Autodesk Inventor part; units mm, degrees
ref_plane "YZ Plane" through (0, 0, 0) normal (1, 0, 0) x (0, 1, 0)
ref_plane "XZ Plane" through (0, 0, 0) normal (0, 1, 0) x (-1, 0, 0)
ref_plane "XY Plane" through (0, 0, 0) normal (0, 0, 1) x (1, 0, 0)
sketch "Sketch1" plane through (0, 0, 0) normal (0, 0, 1) x (1, 0, 0)
  arc A0 (-97, -1740) -> (-70, 0) centre (-11100.8726, -699.0408) ccw
  line L0 (0, 0) -> (-70, 0)
  line L1 (0, -16.732) -> (-68.9524, -16.732) construction
  line L2 (0, -496.732) -> (-49.7243, -496.732) construction
  line L3 (0, -976.732) -> (-51.3615, -976.732) construction
  line L4 (0, -1456.732) -> (-73.8734, -1456.732) construction
  line L5 (-97, -1740) -> (0, -1740)
  line L6 (0, 0) -> (0, -1740)
  line L7 (0, -1730) -> (-10.3553, -1740)
  point P0 (-20, 0)
  dimension "d33" = 50
  dimension "d58" = 480
  dimension "d59" = 480
  dimension "d60" = 480
  dimension "d141" = 1740
  dimension "d148" = 70
  dimension "d149" = 11053
  dimension "d150" = 97
  dimension "d151" = 136
  dimension "d153" = 10
extrude "Plate3" add sketch "Sketch1" along normal blind 3 contours A0 L0 L6 L7 L5
sketch "Sketch3" plane through (-3, 0, 3) normal (1, 0, 0) x (0, 1, 0)
  line L0 (-1730, 0) -> (0, 0)
  line L1 (0, 0) -> (0, 20)
  line L2 (0, 20) -> (-1730, 20)
  line L3 (-1730, 20) -> (-1730, 0)
edge flange "Flange2" height 20 angle 90 thickness 3 bend radius 5 thickness toward (1, 0, 0) relief round relief width 3 relief depth 1.5 edges at (0, -865, 3) wall of the first edge with corners at (-3, -1730, 3) (-3, 0, 3) (-3, 0, -17) (-3, -1730, -17)
bend "Bend2"
corner "Corner2"
sketch "Sketch5" plane through (0, 0, 0) normal (0, 0, 1) x (1, 0, 0)
  line L0 (-8, -1737.7255) -> (-8, 0)
  line L1 (-70, 0) -> (-8, 0)
  arc A0 (-97, -1740) -> (-70, 0) centre (-11100.8726, -699.0408) ccw
  line L2 (0, 0) -> (0, -1730)
  line L3 (0, -198.9) -> (-28, -198.9)
  line L4 (0, -201.1) -> (-3, -201.1)
  line L5 (-3, -1730) -> (-3, 0)
  line L6 (-28, -198.9) -> (-28, -201.1)
  line L7 (0, -608.9) -> (-48.2402, -608.9) construction
  line L8 (0, -1018.9) -> (-52.5018, -1018.9) construction
  line L9 (0, -1428.9) -> (-71.9962, -1428.9) construction
  line L10 (-10.3553, -1740) -> (-97, -1740)
  line L11 (0, -198.9) -> (0, -218.9)
  line L12 (-3, -198.9) -> (-3, -201.1) construction
  line L13 (0, -218.9) -> (-3, -218.9)
  line L14 (-28, -198.9) -> (-59.1939, -198.9) construction
  line L15 (-28, -201.1) -> (-59.0945, -201.1) construction
  line L16 (-3, -201.1) -> (-3, -218.9)
  line L17 (-3, -201.1) -> (-28, -201.1)
  line L18 (-3, -218.9) -> (-8, -218.9)
  line L19 (-8, -1737.7255) -> (-10.3553, -1740)
  line L20 (-4.4351, -201.1) -> (0, -205.5351)
  line L21 (-4.4351, -201.1) -> (1.8371, -201.1) construction
  line L22 (-10.3553, -1740) -> (-10.3553, -1770)
  point P0 (0, 0)
  point P1 (845.25, -380.4205)
  point P2 (848, -380.4205)
  point P3 (-28, -200)
  point P4 (850, -410.4205)
  point P5 (-3, -198.9)
  point P6 (-3, -218.9)
  point P7 (-8, -201.1)
  point P8 (0, -205.5351)
  dimension "d69" = 1730
  dimension "d70" = 2.2
  dimension "d76" = 59.1939
  dimension "d80" = 48.2402
  dimension "d102" = 71.9962
  dimension "d104" = 52.5018
  dimension "d106" = 3
  dimension "d107" = 20
  dimension "d108" = 200
  dimension "d112" = 28
  dimension "d142" = 410
  dimension "d143" = 410
  dimension "d144" = 410
  dimension "d154" = 45
  dimension "d155" = 30
  dimension "d156" = 341.1
extrude "Extrusion2" cut sketch "Sketch5" along normal through all both and the other way through all contours L17 L6 L3 L0 | L0 L3 L5 L17 | L17 L5 L20 | L5 L4 L2 L20 | L3 L2 L4 L5
pattern_linear "Rectangular Pattern3" count 4 spacing 410 along (0, -1, 0) of "Extrusion2"
sketch "Sketch7" plane through (0, 0, 0) normal (0, 0, 1) x (1, 0, 0)
  line L0 (0, 0) -> (0, -198.9)
  line L1 (0, 0) -> (-100, 0)
  line L2 (-100, 0) -> (-100, -940)
  line L3 (-100, -940) -> (0, -940)
  line L4 (0, -940) -> (0, 0)
  line L5 (-100, -1740) -> (0, -1740)
  line L6 (0, -1740) -> (0, -940)
  line L7 (0, -940) -> (-100, -940)
  line L8 (-100, -940) -> (-100, -1740)
  line L9 (-97, -1740) -> (-10.3553, -1740)
  point P0 (-50, -1740)
  dimension "d157" = 100
  dimension "d158" = 940
extrude "Extrusion3" cut sketch "Sketch7" along normal through all both and the other way through all contours L6 L5 L8 L3
equation "\"БОРТ_стрингер_3_высота\" = 59"
equation "\"БОРТ_стрингер_4_высота\" = 48"
equation "\"БОРТ_стрингер_5_высота\" = 53"
equation "\"БОРТ_стрингер_6_высота\" = 72"
properties part number "MSC 347 RIB BOARD" material "Stainless Steel"
Verification items for the finished model (mm, model axes). A direction names the side the tool comes from. Coordinates: 2 decimals unless noted, no trailing zeros. Loops run counter-clockwise (first coordinate to the right, second up) from the corner with the lowest first, then second, coordinate; pieces in that order, holes last. Notation, with made-up numbers: (49.5, 23) - (80.5, 23) arc R25 ccw to (80.5, 42) - close; hole circle Ø5 at (26.5, -8). An arc over 180 degrees is marked (long way). Answer as a JSON object with one key per item and string values.
(1) Cross-section at B-B, the plane x = -18. Record the boundary of the cut face in (y, z), then the cut area to 3 significant figures.
Response:
{"outline": "(-940, 0) - (-611.1, 0) - (-611.1, 3) - (-940, 3) - close; (-608.9, 0) - (-201.1, 0) - (-201.1, 3) - (-608.9, 3) - close; (-198.9, 0) - (0, 0) - (0, 3) - (-198.9, 3) - close", "area": "2,810 mm²"}
(2) Access from +Z, -Z, +X, -X, +Y, -Y to the whole of each face (thin tool, end or side, straight path). Record for faces 4 (the flat face through (-9.8, -608.9, 0.4)), 5 (the flat face through (-29.7, 0, 0.4)).
Response:
{"face 4": "+Z, -Z, +X", "face 5": "+Z, -Z, +X, -X, +Y"}
(3) Scan lines: line 1 along Z through (x, y) = (-26, -359); line 2 along X through (y, z) = (-480.5, -11.75); line 3 along X through (y, z) = (-639.5, -3.75). Record each from-to range of solid material in increasing order.
Response:
{"line 1": "z = 0 to 3", "line 2": "x = -3 to 0", "line 3": "x = -3.16 to -0.1"}
(4) Cross-section at C-C, the plane y = -714. Record the boundary of the cut face in (x, z).
Response:
{"outline": "(-47.88, 0) - (-8, 0) arc R5 cw to (-3, -5) - (-3, -17) - (0, -17) - (0, -5) arc R8 ccw to (-8, 3) - (-47.88, 3) - close"}
(5) Mould release check, pull along Y, two halves, no side actions. Record for faces 1 (the flat face through (-19.8, -940, 0.4)), 2 (the cylindrical face through (-50.39, -463.21, 1.48)), 3 (the flat face through (-33, -463, 0)): pulls with the +Y half, pulls with the -Y half, needs draft (parallel to the pull), parting line crosses it, or undercut.
Response:
{"face 1": "pulls with the -Y half", "face 2": "undercut", "face 3": "needs draft"}
(6) Cross-section at A-A, the plane z = -8.75. Record the boundary of the cut face in (x, y), then the cut area to 3 significant figures.
Response:
{"outline": "(-3, -940) - (0, -940) - (0, -615.54) - (-3, -612.54) - close; (-3, -608.9) - (0, -608.9) - (0, -205.54) - (-3, -202.54) - close; (-3, -198.9) - (0, -198.9) - (0, 0) - (-3, 0) - close", "area": "2,790 mm²"}
(7) Go/stop test with flat-tipped pins: pin 1 Ø3 at (y, z) = (-343, -12) entering from -X; pin 2 Ø0.7 at (y, z) = (-610, 1.5) entering from +X; pin 3 Ø6 at (y, z) = (-262.5, -6) entering from -X. Record where each tip stops, or that it passes through.
Response:
{"pin 1": "stops at x = -3", "pin 2": "stops at x = -28", "pin 3": "stops at x = -3.42"}
